from build123d import *

# Parameters (mm, degrees)
BOSS_EXTRUDE1_DEPTH = 4.699
CUT_EXTRUDE1_REACH  = 116.14
FILLET1_R           = 6.35
FILLET2_R           = 12.7


with BuildPart() as part:
    # Sketch1 → Boss-Extrude1 (new body)
    with BuildSketch(Plane(origin=(0, 0, 0), x_dir=(1, 0, 0), z_dir=(0, 1, 0))):
        with BuildLine():
            Line((0, 25.4), (0, 107.95))
            ThreePointArc((0, 107.95), (18.67009518, 106.323233801), (36.777487633, 101.491964724))
            Line((36.777487633, 101.491964724), (25.4, 85.194189943))
            Line((25.4, 85.194189943), (25.4, 0))
            ThreePointArc((25.4, 0), (17.960512242, -17.960512242), (0, -25.4))
            Line((0, -25.4), (0, -107.95))
            ThreePointArc((0, -107.95), (-18.67009518, -106.323233801), (-36.777487633, -101.491964724))
            Line((-36.777487633, -101.491964724), (-25.4, -85.194189943))
            Line((-25.4, -85.194189943), (-25.4, 0))
            ThreePointArc((-25.4, 0), (-17.960512242, 17.960512242), (0, 25.4))
        make_face()
    extrude(amount=BOSS_EXTRUDE1_DEPTH)

    # Sketch2 → Cut-Extrude1 (cut, up to next)
    with BuildSketch(Plane(origin=(0, 4.699, 0), x_dir=(1, 0, 0), z_dir=(0, 1, 0)), mode=Mode.PRIVATE) as cut_extrude1_sk1:
        Polygon((0, 5.499261314), (-4.7625, 2.749630657), (-4.7625, -2.749630657), (0, -5.499261314), (4.7625, -2.749630657), (4.7625, 2.749630657), align=None)
    cut_extrude1_tool1 = extrude(cut_extrude1_sk1.sketch, amount=-CUT_EXTRUDE1_REACH, mode=Mode.PRIVATE) & part.part
    add(cut_extrude1_tool1.solids().sort_by_distance((0, 4.699, 0))[0], mode=Mode.SUBTRACT)

    # Fillet1
    fillet1_edges = [part.edges().sort_by_distance(p)[0] for p in [
        (0, 2.3495, -25.4),
        (25.4, 2.3495, -85.194189943),
        (0, 2.3495, 25.4),
        (-25.4, 2.3495, 85.194189943),
    ]]
    fillet(fillet1_edges, radius=FILLET1_R)

    # Fillet2
    fillet2_edges = [part.edges().sort_by_distance(p)[0] for p in [
        (0, 2.3495, -107.95),
        (0, 2.3495, 107.95),
    ]]
    fillet(fillet2_edges, radius=FILLET2_R)


solid = part.part
The model under review builds one solid part; all positions refer to its coordinate system, in mm. A direction names the side the tool comes from. Coordinates: 2 decimals unless noted, no trailing zeros. Write each loop counter-clockwise with the first axis right and the second up, starting at its lowest first coordinate (ties: lowest second). Pieces come first, ordered by that corner, then holes. Notation, with made-up numbers: (44.25, -28.75) -> (99.25, -28.75) arc R17 cw to (99.25, -7.75) -> close; hole circle Ø8 at (-22.5, -9.75). An arc over 180 degrees is marked (long way). Answer in a Markdown table with one row per item.
1. Wall thickness on probe 1 along Z at (x, y) = (-4.5, 1.4); probe 2 along X at (y, z) = (2.95, -83); probe 3 along X at (y, z) = (1.05, 66): over which ranges is each line inside the solid? List them lowest first. Write a range as [from, to].
Answers below:
| item | result |
|---|---|
| probe 1 | z = [-25.03, -2.9], [2.9, 104.1] |
| probe 2 | x = [0, 25.4] |
| probe 3 | x = [-25.4, 0] |
2. Clearance check with flat-ended pins moving along their axes: pin 1 Ø2 at (x, y) = (-4.5, 3) entering from +Z; pin 2 Ø1.5 at (x, y) = (-21.5, 1.5) entering from -Z; pin 3 Ø2.5 at (y, z) = (3, 1) entering from +X. State where each tip first meets the part, or that it passes through.
Answers below:
| item | result |
|---|---|
| pin 1 | stops at z = 104.86 |
| pin 2 | stops at z = -14.65 |
| pin 3 | stops at x = 25.4 |
3. We need section A-A, the plane y = 2.9. State the section outline as (x, z) points, and give its area (3 significant figures).
Answers below:
| item | result |
|---|---|
| outline | (-36.78, 101.49) -> (-26.54, 86.83) arc R6.35 cw to (-25.4, 83.2) -> (-25.4, 0) arc R25.4 ccw to (-5.08, -24.89) arc R6.35 cw to (0, -31.11) -> (0, -94.4) arc R12.7 ccw to (14.39, -106.99) arc R107.95 ccw to (36.78, -101.49) -> (26.54, -86.83) arc R6.35 cw to (25.4, -83.2) -> (25.4, 0) arc R25.4 ccw to (5.08, 24.89) arc R6.35 cw to (0, 31.11) -> (0, 94.4) arc R12.7 ccw to (-14.39, 106.99) arc R107.95 ccw to start; hole (-4.76, -2.75) -> (0, -5.5) -> (4.76, -2.75) -> (4.76, 2.75) -> (0, 5.5) -> (-4.76, 2.75) -> close |
| area | 6,520 mm^2 |
4. We need section C-C, the plane x = 19. State the section outline as (y, z) points.
Answers below:
| item | result |
|---|---|
| outline | (0, -106.26) -> (4.7, -106.26) -> (4.7, 16.86) -> (0, 16.86) -> close |
5. For faces 5 (the flat face through (-2.41, 2.38, 4.11)), 6 (the flat face through (0, 2, 62)), 7 (the cylindrical face through (25.575, 2.317, -104.877)), 8 (the flat face through (-25.4, 2, 42)), list the 3-axis set-ups (+Z, -Z, +X, -X, +Y, -Y) from which the entire face can be reached by the end or side of a thin tool; tool diameter is ignored.
Answers below:
| item | result |
|---|---|
| face 5 | +Y, -Y |
| face 6 | +Z, +X, +Y, -Y |
| face 7 | -Z, +X, +Y, -Y |
| face 8 | -Z, -X, +Y, -Y |
6. Draft analysis for pull direction Z (two halves, no side actions). For faces 1 (the cylindrical face through (1.47, 2.382, 27.045)), 2 (the flat face through (4.762, 2, 0)), 3 (the flat face through (-2.348, 2.382, -4.144)), 4 (the flat face through (0, 2, -62)), state which applies: +Z half, -Z half, draft (parallel to the pull), parting line (faces both ways), or undercut.
Answers below:
| item | result |
|---|---|
| face 1 | +Z half |
| face 2 | undercut |
| face 3 | undercut |
| face 4 | draft |
7. We need section B-B, the plane z = 39. State the section outline as (x, y) points.
Answers below:
| item | result |
|---|---|
| outline | (-25.4, 0) -> (0, 0) -> (0, 4.7) -> (-25.4, 4.7) -> close |
